Autodesk Inventor part; units mm, degrees
ref_plane "YZ Plane" through (0, 0, 0) normal (1, 0, 0) x (0, 1, 0)
ref_plane "XZ Plane" through (0, 0, 0) normal (0, 1, 0) x (-1, 0, 0)
ref_plane "XY Plane" through (0, 0, 0) normal (0, 0, 1) x (1, 0, 0)
sketch "Sketch1" plane through (0, 0, 0) normal (1, 0, 0) x (0, 1, 0)
  circle A0 centre (0, 0) radius 27.94
  dimension "d0" = 55.88
extrude "Extrusion1" add sketch "Sketch1" along normal blind 2.54
sketch "Sketch3" plane through (2.54, 0, 0) normal (1, 0, 0) x (0, 0, -1)
  point P0 (0, 0)
  point P1 (15.875, 0)
  dimension "d6" = 15.875
hole "Hole1" at (2.54, 0, -15.875) direction (-1, 0, 0) diameter 3.5052 end through all
pattern_circular "Circular Pattern1" count 6 over 360 about axis through (-10, 0, 0) along (1, 0, 0) of "Hole1"
chamfer "Chamfer1" distance 2.032 angle 18 1 edges at (0, -27.94, 0) measured on face at (0, 4.0768, 2.3537)
sketch "Sketch4" plane through (2.54, 0, 0) normal (1, 0, 0) x (0, 0, -1)
  circle A0 centre (0, 0) radius 10.16
  dimension "d20" = 20.32
extrude "Extrusion3" cut sketch "Sketch4" against normal through all
properties part number "ScorpioSprocketFlange" material "ABS Plastic"
Work out the finished part from the listing and answer in its coordinate system (mm). Coordinates: 2 decimals unless noted, no trailing zeros. Write each loop counter-clockwise with the first axis right and the second up, starting at its lowest first coordinate (ties: lowest second). Pieces come first, ordered by that corner, then holes. Notation, with made-up numbers: (48, 35) - (96, 35) arc R32 cw to (96, 71) - close; hole circle Ø9 at (-20.5, 26.25). An arc over 180 degrees is marked (long way). One line per question, with ' | ' between items.
1) The mould has two halves that part along Z. Classify faces 1 (the face through (1.25, -14.81, -9.33)), 2 (the face through (1.25, 14.81, 9.33)), 3 (the face through (1.59, -3.64, -27.7)), 4 (the face through (2.54, 12, 0)): +Z half, -Z half, draft (parallel to the pull), parting line (faces both ways), or undercut.
Checks:
face 1: undercut | face 2: undercut | face 3: parting line | face 4: draft
2) Find section C-C, the plane x = 2.15. Determine the outline of the cut face in (y, z) (1 decimal), and give its area (3 significant figures).
Checks:
outline: circle Ø55.9 at (0, 0); hole circle Ø3.5 at (-13.7, -7.9); hole circle Ø3.5 at (-13.7, 7.9); hole circle Ø20.3 at (0, 0); hole circle Ø3.5 at (0, -15.9); hole circle Ø3.5 at (0, 15.9); hole circle Ø3.5 at (13.7, -7.9); hole circle Ø3.5 at (13.7, 7.9) | area: 2,070 mm2
3) Find section B-B, the plane y = 0. Determine the outline of the cut face in (x, z), and give its area (3 significant figures).
Checks:
outline: (0, -25.91) - (0.66, -27.94) - (2.54, -27.94) - (2.54, -17.63) - (0, -17.63) - close; (0, -14.12) - (2.54, -14.12) - (2.54, -10.16) - (0, -10.16) - close; (0, 10.16) - (2.54, 10.16) - (2.54, 14.12) - (0, 14.12) - close; (0, 17.63) - (2.54, 17.63) - (2.54, 27.94) - (0.66, 27.94) - (0, 25.91) - close | area: 71.2 mm2
4) Consider probe 1 along Y at (x, z) = (1, 8.5); probe 2 along Y at (x, z) = (1.35, 7); probe 3 along Z at (x, y) = (2, -8). Determine where each line is inside the solid, lowest interval first. Write a range as [from, to].
Checks:
probe 1: [-26.62, -15.41], [-12.09, -5.57], [5.57, 12.09], [15.41, 26.62] | probe 2: [-27.05, -15.23], [-12.27, -7.36], [7.36, 12.27], [15.23, 27.05] | probe 3: [-26.77, -6.26], [6.26, 26.77]
5) Find section D-D, the plane z = 7.5. Give the number of separate pieces and of enclosed holes in the cut face, and give its area (3 significant figures).
Checks:
separate pieces: 4 | enclosed holes: 0 | area: 83.3 mm2
6) Find section A-A, the plane z = 0. Determine the outline of the cut face in (x, y).
Checks:
outline: (0, -25.91) - (0.66, -27.94) - (2.54, -27.94) - (2.54, -10.16) - (0, -10.16) - close; (0, 10.16) - (2.54, 10.16) - (2.54, 27.94) - (0.66, 27.94) - (0, 25.91) - close
7) Flat-ended cylindrical pins translate along their axes: P1, Ø3, axis at y = -13.75, z = -7.94, coming from the -X side; P2, Ø4, axis at y = 13.75, z = 7.94, coming from the +X side; P3, Ø1, axis at x = 1.5, z = -17, coming from the +Y side. Find the tip coordinate at first contact, or state that the pin passes through.
Checks:
P1: through | P2: x = 2.54 | P3: y = 22.55
